```python
from build123d import *

# Parameters (mm, degrees)
SKETCH1_W               = 10
SKETCH1_H               = 57.15
SKETCH1_W_2             = 95.25
SKETCH1_H_2             = 6
BOSS_EXTRUDE1_DEPTH     = 25.4
RIB1_REACH              = 82.817
SKETCH2_WALL_W          = 258.734123662
SKETCH2_WALL_H          = 10
CHAMFER2_SIZE           = 5
CHAMFER3_SIZE           = 5
CUT_EXTRUDE1_DEPTH      = 79.60930686
CUT_EXTRUDE1_DEPTH_BACK = 79.60930686
SKETCH3_R               = 3
SKETCH4_R               = 7.5
CUT_EXTRUDE2_DEPTH      = 79.60930686
FILLET1_R               = 10
FILLET2_R               = 10
CUT_EXTRUDE3_REACH      = 109.381
SKETCH5_R               = 3
FILLET3_R               = 1


with BuildPart() as part:
    # Sketch1 → Boss-Extrude1 (new, symmetric)
    with BuildSketch(Plane.XY):
        with Locations((-42.625, 31.575)):
            Rectangle(SKETCH1_W, SKETCH1_H)
        Rectangle(SKETCH1_W_2, SKETCH1_H_2)
    extrude(amount=BOSS_EXTRUDE1_DEPTH, both=True)

    # Sketch2 wall → Rib1 (add, up to next)
    with BuildSketch(Plane(origin=(5, 24.075, 0), x_dir=(0.896416143278, -0.443213377586, 0), z_dir=(0.443213377586, 0.896416143278, 0)), mode=Mode.PRIVATE) as rib1_sk1:
        Rectangle(SKETCH2_WALL_W, SKETCH2_WALL_H)
    rib1_tool1 = extrude(rib1_sk1.sketch, amount=-RIB1_REACH, mode=Mode.PRIVATE) - part.part
    add(rib1_tool1.solids().sort_by_distance((5, 24.075, 0))[0])

    # Chamfer2
    chamfer2_edges = [part.edges().sort_by_distance(p)[0] for p in [
        (-37.625, 24.075, 5),
        (5, 3, 5),
    ]]
    chamfer(chamfer2_edges, length=CHAMFER2_SIZE)

    # Chamfer3
    # the kernel refuses this chamfer: 5 mm, written as the material it adds along each edge
    with BuildSketch(Plane(origin=(-37.625, 58.00841494, -5), x_dir=(-0.027495876610586317, 0, -0.9996219169112968), z_dir=(0, -1, 0))) as chamfer3_piece_1_section:
        Polygon((CHAMFER3_SIZE * 0.999621916911, CHAMFER3_SIZE * 0.0274958766106), (-CHAMFER3_SIZE * 0.0274958766106, CHAMFER3_SIZE * 0.999621916911), (0, 0), align=None)
    chamfer3_piece_1 = extrude(amount=55.00841494, mode=Mode.PRIVATE)
    chamfer3_piece_1 = split(chamfer3_piece_1, bisect_by=Plane(origin=(-27.763842546, 40.274366139, -6.674975075), z_dir=(-0.4432133775858684, -0.8964161432777338, 0)), keep=Keep.TOP, mode=Mode.PRIVATE)
    add(chamfer3_piece_1)
    with BuildSketch(Plane(origin=(60.48341494, 3, -5), x_dir=(0, 0.9996219169112968, 0.027495876610586244), z_dir=(-1, 0, 0))) as chamfer3_piece_2_section:
        Polygon((CHAMFER3_SIZE * 0.999621916911, CHAMFER3_SIZE * 0.0274958766106), (-CHAMFER3_SIZE * 0.0274958766106, CHAMFER3_SIZE * 0.999621916911), (0, 0), align=None)
    chamfer3_piece_2 = extrude(amount=110.96682988, mode=Mode.PRIVATE)
    chamfer3_piece_2 = split(chamfer3_piece_2, bisect_by=Plane(origin=(-47.625, 4.632358995, -6.683820502), z_dir=(1, 0, 0)), keep=Keep.TOP, mode=Mode.PRIVATE)
    chamfer3_piece_2 = split(chamfer3_piece_2, bisect_by=Plane(origin=(11.398148356, 20.911575329, -6.683820502), z_dir=(-0.4432133775858684, -0.8964161432777338, 0)), keep=Keep.TOP, mode=Mode.PRIVATE)
    add(chamfer3_piece_2)

    # Sketch3 → Cut-Extrude1 (cut, two sides: drawn at the far end of the back side and taken through both)
    with BuildSketch(Plane(origin=(0, 3, 0), x_dir=(1, 0, 0), z_dir=(0, 1, 0)).offset(-CUT_EXTRUDE1_DEPTH_BACK)):
        with Locations(Location((24.925, 12.7, 0), (0, 0, 270))):
            Circle(SKETCH3_R)
        with Locations(Location((24.925, -12.7, 0), (0, 0, 270))):
            Circle(SKETCH3_R)
        with Locations(Location((37.625, -12.7, 0), (0, 0, 270))):
            Circle(SKETCH3_R)
        with Locations(Location((37.625, 12.7, 0), (0, 0, 270))):
            Circle(SKETCH3_R)
    extrude(amount=CUT_EXTRUDE1_DEPTH + CUT_EXTRUDE1_DEPTH_BACK, mode=Mode.SUBTRACT)

    # Sketch4 → Cut-Extrude2 (cut, through all)
    with BuildSketch(Plane(origin=(0, 3, 0), x_dir=(1, 0, 0), z_dir=(0, 1, 0))):
        with BuildLine():
            ThreePointArc((31.275, -16.690927211), (39.701655966, -19.906767653), (45.125, -12.7))
            ThreePointArc((45.125, -12.7), (44.998213921, -11.326786079), (44.622142274, -10))
            Line((44.622142274, -10), (38.932669683, -10))
            ThreePointArc((38.932669683, -10), (37.625, -15.7), (36.317330317, -10))
            Line((36.317330317, -10), (31.922142274, -10))
            ThreePointArc((31.922142274, -10), (32.298213921, -11.326786079), (32.425, -12.7))
            ThreePointArc((32.425, -12.7), (32.131767653, -14.776655966), (31.275, -16.690927211))
        make_face()
        with BuildLine():
            Line((38.932669683, -10), (44.622142274, -10))
            ThreePointArc((44.622142274, -10), (38.347026001, -5.234835671), (31.275, -8.709072789))
            ThreePointArc((31.275, -8.709072789), (31.629712894, -9.338925021), (31.922142274, -10))
            Line((31.922142274, -10), (36.317330317, -10))
            ThreePointArc((36.317330317, -10), (37.625, -15.7), (38.932669683, -10))
        make_face()
        with BuildLine():
            ThreePointArc((17.927857726, -10), (21.563925021, -19.404712894), (31.275, -16.690927211))
            ThreePointArc((31.275, -16.690927211), (30.159835671, -13.422026001), (30.627857726, -10))
            Line((30.627857726, -10), (26.232669683, -10))
            ThreePointArc((26.232669683, -10), (24.925, -15.7), (23.617330317, -10))
            Line((23.617330317, -10), (17.927857726, -10))
        make_face()
        with BuildLine():
            ThreePointArc((30.627857726, -10), (30.920287106, -9.338925021), (31.275, -8.709072789))
            ThreePointArc((31.275, -8.709072789), (24.202973999, -5.234835671), (17.927857726, -10))
            Line((17.927857726, -10), (23.617330317, -10))
            ThreePointArc((23.617330317, -10), (24.925, -15.7), (26.232669683, -10))
            Line((26.232669683, -10), (30.627857726, -10))
        make_face()
        with BuildLine():
            ThreePointArc((30.627857726, -10), (30.159835671, -13.422026001), (31.275, -16.690927211))
            ThreePointArc((31.275, -16.690927211), (32.131767653, -14.776655966), (32.425, -12.7))
            ThreePointArc((32.425, -12.7), (32.298213921, -11.326786079), (31.922142274, -10))
            Line((31.922142274, -10), (30.627857726, -10))
        make_face()
        with BuildLine():
            ThreePointArc((31.922142274, -10), (31.629712894, -9.338925021), (31.275, -8.709072789))
            ThreePointArc((31.275, -8.709072789), (30.920287106, -9.338925021), (30.627857726, -10))
            Line((30.627857726, -10), (31.922142274, -10))
        make_face()
        with Locations((24.925, 12.7)):
            Circle(SKETCH4_R)
        with Locations((37.625, 12.7)):
            Circle(SKETCH4_R)
    extrude(amount=CUT_EXTRUDE2_DEPTH, mode=Mode.SUBTRACT)

    # Fillet1
    fillet1_edges = [part.edges().sort_by_distance(p)[0] for p in [
        (47.625, 0, 25.4),
        (47.625, 0, -25.4),
    ]]
    fillet(fillet1_edges, radius=FILLET1_R)

    # Fillet2
    fillet2_edges = [part.edges().sort_by_distance(p)[0] for p in [
        (-42.625, 60.15, 25.4),
        (-42.625, 60.15, -25.4),
    ]]
    fillet(fillet2_edges, radius=FILLET2_R)

    # Sketch5 → Cut-Extrude3 (cut, up to next)
    with BuildSketch(Plane(origin=(-37.625, 0, 0), x_dir=(0, 0, -1), z_dir=(1, 0, 0)), mode=Mode.PRIVATE) as cut_extrude3_sk1:
        with Locations(Location((-17.5, 50.15, 0), (0, 0, 90))):
            Circle(SKETCH5_R)
    cut_extrude3_tool1 = extrude(cut_extrude3_sk1.sketch, amount=-CUT_EXTRUDE3_REACH, mode=Mode.PRIVATE) & part.part
    # Sketch5 → Cut-Extrude3 (cut, up to next)
    with BuildSketch(Plane(origin=(-37.625, 0, 0), x_dir=(0, 0, -1), z_dir=(1, 0, 0)), mode=Mode.PRIVATE) as cut_extrude3_sk2:
        with Locations(Location((17.5, 50.15, 0), (0, 0, 90))):
            Circle(SKETCH5_R)
    cut_extrude3_tool2 = extrude(cut_extrude3_sk2.sketch, amount=-CUT_EXTRUDE3_REACH, mode=Mode.PRIVATE) & part.part
    # Sketch5 → Cut-Extrude3 (cut, up to next)
    with BuildSketch(Plane(origin=(-37.625, 0, 0), x_dir=(0, 0, -1), z_dir=(1, 0, 0)), mode=Mode.PRIVATE) as cut_extrude3_sk3:
        with Locations(Location((17.5, 30.15, 0), (0, 0, 90))):
            Circle(SKETCH5_R)
    cut_extrude3_tool3 = extrude(cut_extrude3_sk3.sketch, amount=-CUT_EXTRUDE3_REACH, mode=Mode.PRIVATE) & part.part
    # Sketch5 → Cut-Extrude3 (cut, up to next)
    with BuildSketch(Plane(origin=(-37.625, 0, 0), x_dir=(0, 0, -1), z_dir=(1, 0, 0)), mode=Mode.PRIVATE) as cut_extrude3_sk4:
        with Locations(Location((-17.5, 30.15, 0), (0, 0, 90))):
            Circle(SKETCH5_R)
    cut_extrude3_tool4 = extrude(cut_extrude3_sk4.sketch, amount=-CUT_EXTRUDE3_REACH, mode=Mode.PRIVATE) & part.part
    # Sketch5 → Cut-Extrude3 (cut, up to next)
    with BuildSketch(Plane(origin=(-37.625, 0, 0), x_dir=(0, 0, -1), z_dir=(1, 0, 0)), mode=Mode.PRIVATE) as cut_extrude3_sk5:
        with Locations(Location((-17.5, 10.15, 0), (0, 0, 90))):
            Circle(SKETCH5_R)
    cut_extrude3_tool5 = extrude(cut_extrude3_sk5.sketch, amount=-CUT_EXTRUDE3_REACH, mode=Mode.PRIVATE) & part.part
    # Sketch5 → Cut-Extrude3 (cut, up to next)
    with BuildSketch(Plane(origin=(-37.625, 0, 0), x_dir=(0, 0, -1), z_dir=(1, 0, 0)), mode=Mode.PRIVATE) as cut_extrude3_sk6:
        with Locations(Location((17.5, 10.15, 0), (0, 0, 90))):
            Circle(SKETCH5_R)
    cut_extrude3_tool6 = extrude(cut_extrude3_sk6.sketch, amount=-CUT_EXTRUDE3_REACH, mode=Mode.PRIVATE) & part.part
    add(cut_extrude3_tool1.solids().sort_by_distance((-37.625, 50.15, 17.5))[0], mode=Mode.SUBTRACT)
    add(cut_extrude3_tool2.solids().sort_by_distance((-37.625, 50.15, -17.5))[0], mode=Mode.SUBTRACT)
    add(cut_extrude3_tool3.solids().sort_by_distance((-37.625, 30.15, -17.5))[0], mode=Mode.SUBTRACT)
    add(cut_extrude3_tool4.solids().sort_by_distance((-37.625, 30.15, 17.5))[0], mode=Mode.SUBTRACT)
    add(cut_extrude3_tool5.solids().sort_by_distance((-37.625, 10.15, 17.5))[0], mode=Mode.SUBTRACT)
    add(cut_extrude3_tool6.solids().sort_by_distance((-37.625, 10.15, -17.5))[0], mode=Mode.SUBTRACT)

    # Fillet3
    # the kernel refuses this fillet: 1 mm, written as the material it takes off along each edge
    with BuildSketch(Plane(origin=(31.275, 7.401030704, -8.709072789), x_dir=(-0.6005096173498707, 0, 0.7996175332434325), z_dir=(0, -1, 0))) as fillet3_piece_1:
        with BuildLine():
            CenterArc((1.326977491, -0.996554868), FILLET3_R, 94.7573526, 96.67248475)
            ThreePointArc((0.346809381, -1.194722667), (0.198218842, -0.590158172), (0, 0))
            ThreePointArc((0, 0), (0.622020699, -0.025838492), (1.244041397, 0))
        make_face()
    extrude(amount=4.401030704, mode=Mode.SUBTRACT)
    with BuildSketch(Plane(origin=(31.275, 3, 8.709072789), x_dir=(0.6005096173499003, 0, -0.7996175332434102), z_dir=(0, 1, 0))) as fillet3_piece_2:
        with BuildLine():
            CenterArc((1.326977491, 0.996554868), FILLET3_R, 168.570162651, 96.67248475)
            ThreePointArc((0.346809381, 1.194722667), (0.198218842, 0.590158172), (0, 0))
            ThreePointArc((0, 0), (0.622020699, 0.025838492), (1.244041397, 0))
        make_face()
    extrude(amount=4.401030704, mode=Mode.SUBTRACT)


solid = part.part
```
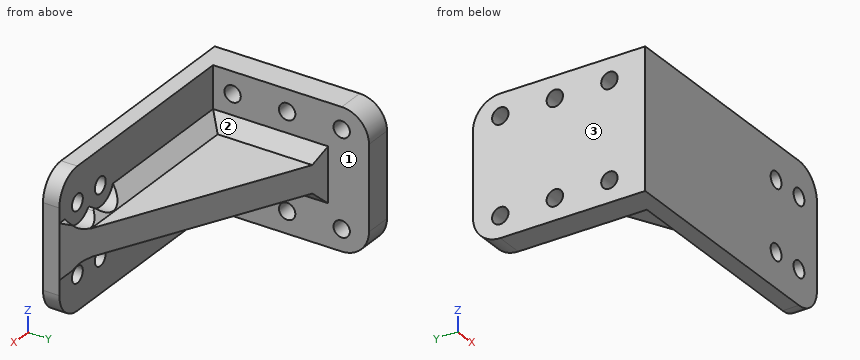
Part model, mm, in its own coordinate system. Face numbers are marked on the shaded views. A direction names the side the tool comes from. Round coordinates to 2 decimals unless told otherwise and drop trailing zeros. Order: outer loops, then holes, each group sorted by start corner. A loop starts at its lowest first (then second) coordinate and runs counter-clockwise, first axis right, second up. Notation, with made-up numbers: M -7,70 L 34,70 A26 cw 34,101 Z; hole C 87.5,17.25 d9. An arc over 180 degrees is marked long. Put each result on its own line as item: value. Start each with the question number.
1. Drop flat-ended pins along their axis: pin 1 (16 mm diameter, centred on x = 15.5, z = 16.5, fed in from +Y); pin 2 (7 mm diameter, centred on x = 37.625, z = -12.7, fed in from +Y); pin 3 (3.5 mm diameter, centred on y = 50.15, z = 17.5, fed in from +X); pin 4 (7 mm diameter, centred on y = 10.15, z = 17.5, fed in from +X) (3 decimals). Give the stop position or say it passes through.
2. Slice it at C-C on x = 4.5. List the corners of the cut face in (y, z).
3. Slice it at B-B on y = 32. List the corners of the cut face in (x, z) (3 decimals), then the cut area to 3 significant figures.
4. Slice it at D-D on y = 14.5. List the corners of the cut face in (x, z) (3 decimals), then the cut area to 3 significant figures.
5. Slice it at A-A on z = -12.7. List the corners of the cut face in (x, y) (3 decimals).
6. Tool access for the marked faces 1, 2 and 3: list every direction of +Z, -Z, +X, -X, +Y, -Y with a clear straight run to the whole face (end or side of a thin tool).
7. Drill centre lines: probe 1 along Z at (x, y) = (-40.75, 30.15); probe 2 along X at (y, z) = (1.25, 12.7) (3 decimals); probe 3 along Z at (x, y) = (-15.5, 19). Where is each one in solid material? Low to high. Write a range as [from, to].
Findings:
1. pin 1: y = 4.5
1. pin 2: y = 3
1. pin 3: through
1. pin 4: x = -37.625
2. outline: M -3,-25.4 L 3,-25.4 L 3,-10 L 8,-5 L 24.32,-5 L 24.32,5 L 8,5 L 3,10 L 3,25.4 L -3,25.4 Z
3. outline: M -47.625,-25.4 L -37.625,-25.4 L -37.625,-19.862 L -47.625,-19.862 Z; M -47.625,-15.138 L -37.625,-15.138 L -37.625,-10 L -32.625,-5 L -11.029,-5 L -11.029,5 L -32.625,5 L -37.625,10 L -37.625,15.138 L -47.625,15.138 Z; M -47.625,19.862 L -37.625,19.862 L -37.625,25.4 L -47.625,25.4 Z
3. area: 704 mm2
4. outline: M -47.625,-25.4 L -37.625,-25.4 L -37.625,-10 L -32.625,-5 L 24.366,-5 L 24.366,5 L -32.625,5 L -37.625,10 L -37.625,25.4 L -47.625,25.4 Z
4. area: 1,150 mm2
5. outline: M -47.625,-3 L 21.925,-3 L 21.925,3 L -37.625,3 L -37.625,60.15 L -47.625,60.15 Z; M 27.925,-3 L 34.625,-3 L 34.625,3 L 27.925,3 Z; M 40.625,-3 L 47.625,-3 L 47.625,3 L 40.625,3 Z
6. face 1: +X, +Y
6. face 2: +Z, +X, +Y
6. face 3: +Z, -Z, -X, +Y, -Y
7. probe 1: [-25.4, -20.5], [-14.5, 14.5], [20.5, 25.4]
7. probe 2: [-47.625, 21.925], [27.925, 34.625], [40.625, 47.625]
7. probe 3: [-5, 5]
